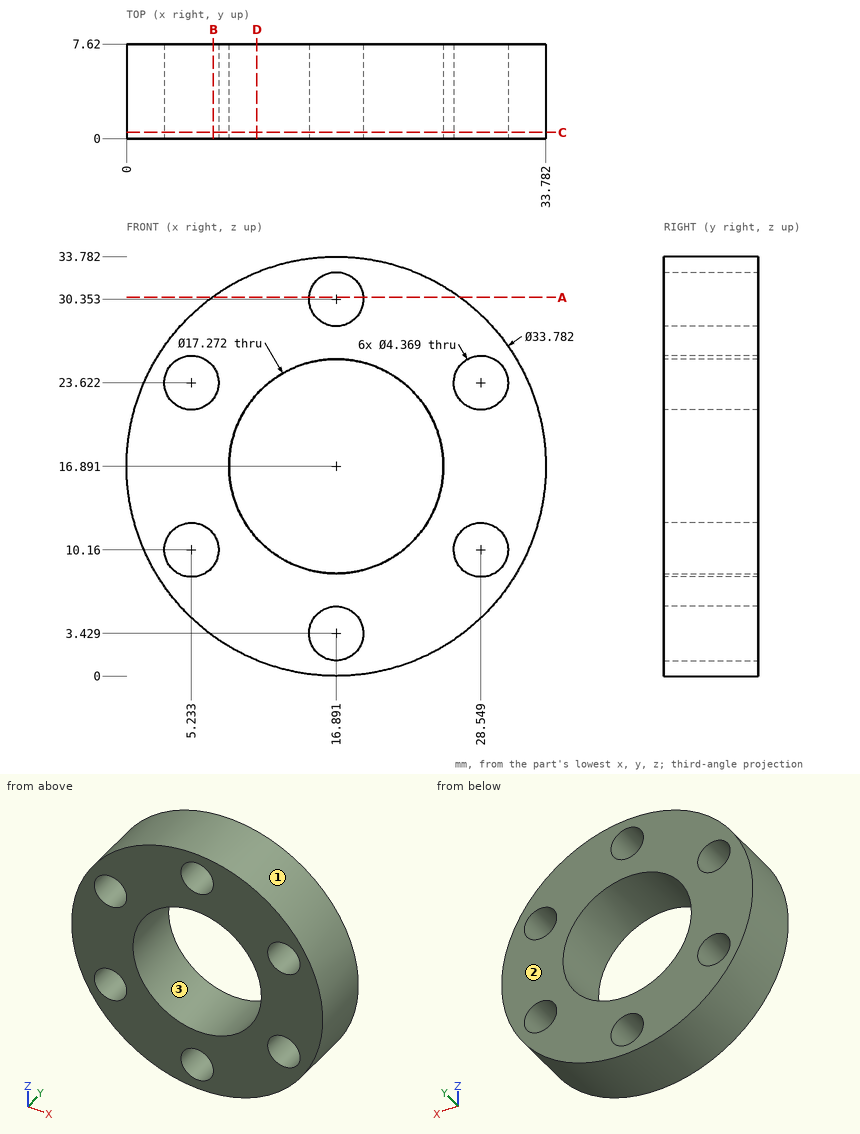
Design review of the part shown in the three views and the two pictorial views. Dimensions are in mm from the part's minimum x, y and z. Round coordinates to 2 decimals unless told otherwise and drop trailing zeros. Loops run counter-clockwise (first coordinate to the right, second up) from the corner with the lowest first, then second, coordinate; pieces in that order, holes last. Notation, with made-up numbers: M -12.75,-1 L 45.25,-1 A7 cw 45.25,8 Z; hole C -7,45 d7. An arc over 180 degrees is marked long. Put each result on its own line as item: value.
Q1. To check wall thickness, follow L1, parallel to Z at x = 30, y = 3.25 (1 decimal); L2, parallel to Z at x = 4.5, y = 2.5 (1 decimal); L3, parallel to X at y = 2.5, z = 24 (1 decimal). State the ranges of each line that lie inside material, in increasing order.
Result set:
L1: z = 6.2 to 8.5, 11.8 to 22, 25.3 to 27.5
L2: z = 5.4 to 8.1, 12.2 to 21.6, 25.7 to 28.4
L3: x = 1.6 to 3.1, 7.4 to 12, 21.8 to 26.4, 30.7 to 32.2
Q2. Consider section D-D, the plane x = 10.5. Give the boundary of the cut face in (y, z) (1 decimal).
Result set:
outline: M 0,1.3 L 7.6,1.3 L 7.6,11.1 L 0,11.1 Z; M 0,22.7 L 7.6,22.7 L 7.6,32.5 L 0,32.5 Z
Q3. Consider section A-A, the plane z = 30.5. Give the boundary of the cut face in (x, y).
Result set:
outline: M 6.89,0 L 14.71,0 L 14.71,7.62 L 6.89,7.62 Z; M 19.07,0 L 26.9,0 L 26.9,7.62 L 19.07,7.62 Z
Q4. Consider section B-B, the plane x = 7. Give the boundary of the cut face in (y, z) (1 decimal).
Result set:
outline: M 0,3.2 L 7.6,3.2 L 7.6,8.9 L 0,8.9 Z; M 0,11.4 L 7.6,11.4 L 7.6,22.3 L 0,22.3 Z; M 0,24.9 L 7.6,24.9 L 7.6,30.6 L 0,30.6 Z
Q5. Mouldability with a two-part tool opening along X and no side actions: class the marked faces 1, 2 and 3 as released by +X, released by -X, zero draft, split by the parting line, or undercut.
Result set:
face 1: split by the parting line
face 2: zero draft
face 3: undercut
Q6. For pin 1 (15.5 mm diameter, centred on x = 16.891, z = 16.891, fed in from -Y); pin 2 (5.5 mm diameter, centred on x = 16.891, z = 30.353, fed in from +Y); pin 3 (4 mm diameter, centred on y = 1.5, z = 25, fed in from +X); pin 4 (2 mm diameter, centred on y = 4, z = 26.5, fed in from +X), all flat-tipped, find the tip position at first contact; note any pin that passes through.
Result set:
pin 1: passes through
pin 2: stops at y = 7.62
pin 3: stops at x = 32.64
pin 4: stops at x = 31.42
Q7. Consider section C-C, the plane y = 0.5. Count the separate pieces of the cut face and the enclosed holes in it, then the cut area to 3 significant figures.
Result set:
separate pieces: 1
enclosed holes: 7
area: 572 mm²
